Autodesk Inventor part; units mm, degrees
ref_plane "YZ Plane" through (0, 0, 0) normal (1, 0, 0) x (0, 1, 0)
ref_plane "XZ Plane" through (0, 0, 0) normal (0, 1, 0) x (-1, 0, 0)
ref_plane "XY Plane" through (0, 0, 0) normal (0, 0, 1) x (1, 0, 0)
sketch "Sketch1" plane through (0, 0, 0) normal (0, 1, 0) x (-1, 0, 0)
  circle A0 centre (0, 0) radius 35
  circle A1 centre (35, 0) radius 4
  circle A2 centre (28.3156, 20.5725) radius 4
  circle A3 centre (10.8156, 33.287) radius 4
  circle A4 centre (-10.8156, 33.287) radius 4
  circle A5 centre (-28.3156, 20.5725) radius 4
  circle A6 centre (-35, 0) radius 4
  circle A7 centre (-28.3156, -20.5725) radius 4
  circle A8 centre (-10.8156, -33.287) radius 4
  circle A9 centre (10.8156, -33.287) radius 4
  circle A10 centre (28.3156, -20.5725) radius 4
  circle A11 centre (0, 0) radius 39
  point P0 (-25.7834, 23.6689)
  point P1 (-14.543, 31.8355)
  point P2 (-6.947, 34.3036)
  point P3 (6.947, 34.3036)
  point P4 (14.543, 31.8355)
  point P5 (25.7834, 23.6689)
  point P6 (30.478, 17.2074)
  point P7 (34.7714, 3.9935)
  point P8 (34.7714, -3.9935)
  point P9 (30.478, -17.2074)
  point P10 (25.7834, -23.6689)
  point P11 (14.543, -31.8355)
  point P12 (6.947, -34.3036)
  point P13 (-6.947, -34.3036)
  point P14 (-14.543, -31.8355)
  point P15 (-25.7834, -23.6689)
  point P16 (-30.478, -17.2074)
  point P17 (-34.7714, -3.9935)
  point P18 (-34.7714, 3.9935)
  point P19 (-30.478, 17.2074)
  dimension "d1" = 70
  dimension "d2" = 8
  dimension "d5" = 360
  dimension "d7" = 78
extrude "Extrusion1" add sketch "Sketch1" against normal blind 5
extrude "Extrusion2" add sketch "Sketch1" along normal blind 10 contours A0 A1 | A0 A1 | A0 A2 A11 A1 | A1 A11 A10 A0 | A2 A0 | A0 A2 | A10 A0 | A0 A10 | A0 A3 A11 A2 | A11 A9 A0 A10 | A3 A0 | A0 A3 | A3 A0 A4 A11 | A11 A8 A0 A9 | A9 A0 | A0 A9 | A4 A0 | A4 A0 A5 A11 | A11 A7 A0 A8 | A8 A0 | A4 A0 | A5 A0 | A5 A0 A6 A11 | A0 A8 | A11 A6 A0 A7 | A7 A0 | A5 A0 | A6 A0 | A0 A7 | A6 A0
sketch "Sketch2" plane through (0, 0, 0) normal (0, 1, 0) x (1, 0, 0)
  circle A0 centre (0, 0) radius 5
  dimension "d12" = 10
extrude "Extrusion3" cut sketch "Sketch2" against normal blind 10
sketch "Sketch3" plane through (0, -5, 0) normal (0, -1, 0) x (1, 0, 0)
  circle A0 centre (0, 0) radius 24
  dimension "d18" = 48
extrude "Extrusion4" cut sketch "Sketch3" against normal blind 10
properties part number "ring"
Design review of the part built by this model. Coordinates are the model's own, in mm. A direction names the side the tool comes from. Coordinates: 2 decimals unless noted, no trailing zeros. Loops run counter-clockwise (first coordinate to the right, second up) from the corner with the lowest first, then second, coordinate; pieces in that order, holes last. Notation, with made-up numbers: M 27.5,44.25 L 76.5,44.25 A24 cw 76.5,64.25 Z; hole C 19.25,-3 d2. An arc over 180 degrees is marked long. Answer as CSV lines item,"result".
Item 1: For P1, Ø6, axis at x = -21.5, y = 7.5, coming from the +Z side; P2, Ø6, axis at x = -11, y = 7.5, coming from the +Z side; P3, Ø4, axis at y = 3.5, z = -30, coming from the -X side, all flat-tipped, find the tip position at first contact; note any pin that passes through.
Answer list:
P1,"z = 34.33"
P2,"z = 38.17"
P3,"x = -27.15"
Item 2: Add section B-B on x = 0. State the section outline as (y, z) points.
Answer list:
outline,"M -5,-39 L 10,-39 L 10,-35 L 0,-35 L 0,-24 L -5,-24 Z; M -5,24 L 0,24 L 0,35 L 10,35 L 10,39 L -5,39 Z"
Item 3: Machinability: for faces 1 (the face through (-23.977, -2.535, 1.055)), 2 (the face through (20.493, 4.93, -28.373)), which of the approach directions +Z, -Z, +X, -X, +Y, -Y give a long, thin tool a straight path to every point of the face, cutting with its end or side? Answer none if there is none.
Answer list:
face 1,"+Y, -Y"
face 2,"+Y"
Item 4: Add section D-D on x = 33. State the section outline as (y, z) points.
Answer list:
outline,"M -5,-20.78 L 10,-20.78 L 10,-11.66 L 0,-11.66 L 0,-3.46 L 10,-3.46 L 10,3.46 L 0,3.46 L 0,11.66 L 10,11.66 L 10,20.78 L -5,20.78 Z"
Item 5: Add section A-A on z = 0. State the section outline as (x, y) points.
Answer list:
outline,"M -39,-5 L -24,-5 L -24,0 L -31,0 L -31,10 L -39,10 Z; M 24,-5 L 39,-5 L 39,10 L 31,10 L 31,0 L 24,0 Z"
Item 6: The part is to be moulded in two halves that separate along Z. For faces 3 (the face through (25.13, 4.93, -18.153)), 4 (the face through (5.077, 2.395, -38.668)), 5 (the face through (-17, -5, 18)), say which applies: pulls with the +Z half, pulls with the -Z half, needs draft (parallel to the pull), parting line crosses it, or undercut.
Answer list:
face 3,"undercut"
face 4,"parting line crosses it"
face 5,"needs draft"
Item 7: Add section C-C on y = 1.75. State the section outline as (x, z) points.
Answer list:
outline,"C 0,0 d78; hole M -34.77,-3.99 A35 ccw -30.48,-17.21 A4 cw -25.78,-23.67 A35 ccw -14.54,-31.84 A4 cw -6.95,-34.3 A35 ccw 6.95,-34.3 A4 cw 14.54,-31.84 A35 ccw 25.78,-23.67 A4 cw 30.48,-17.21 A35 ccw 34.77,-3.99 A4 cw 34.77,3.99 A35 ccw 30.48,17.21 A4 cw 25.78,23.67 A35 ccw 14.54,31.84 A4 cw 6.95,34.3 A35 ccw -6.95,34.3 A4 cw -14.54,31.84 A35 ccw -25.78,23.67 A4 cw -30.48,17.21 A35 ccw -34.77,3.99 A4 cw Z"
Item 8: For probe 1 along Z at (x, y) = (0, -2.55); probe 2 along Z at (x, y) = (-1, 5.25); probe 3 along X at (y, z) = (8.5, -30) (3 decimals), list the stretches that pass through material, from the lowest coordinate up.
Answer list:
probe 1,"-39 to -24, 24 to 39"
probe 2,"-38.99 to -34.99, 34.99 to 38.99"
probe 3,"-24.92 to -18.028, -13.095 to -8.536, 8.536 to 13.095, 18.028 to 24.92"
